Here's how the part is built. I have some questions about the finished solid (model axes, mm). Face numbers are marked on the shaded views. A direction names the side the tool comes from. Give positions to 0.01 mm unless a question says otherwise; leave off trailing zeros. Write each loop counter-clockwise with the first axis right and the second up, starting at its lowest first coordinate (ties: lowest second). Pieces come first, ordered by that corner, then holes. Notation, with made-up numbers: (19.25, 71.5) - (57.25, 71.5) arc R21 ccw to (57.25, 99.5) - close; hole circle Ø10 at (-32.75, -13). An arc over 180 degrees is marked (long way). Use a Markdown table: item, result.
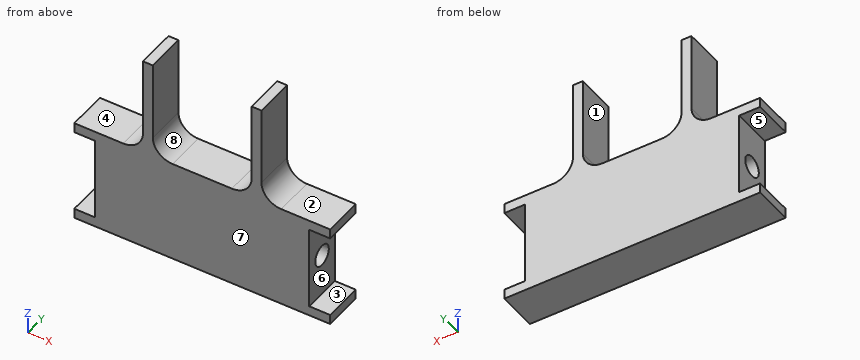
```python
from build123d import *

# Parameters (mm, degrees)
BOSS_EXTRUDE1_DEPTH = 12
SKETCH2_R           = 3.175
CUT_EXTRUDE1_DEPTH  = 79.871937341
SKETCH3_W           = 3
SKETCH3_H           = 12
BOSS_EXTRUDE2_DEPTH = 30
FILLET1_R           = 6


with BuildPart() as part:
    # Sketch1 → Boss-Extrude1 (new body)
    with BuildSketch(Plane(origin=(0, 0, 0), x_dir=(1, 0, 0), z_dir=(0, 1, 0))):
        Polygon((0, 0), (0, 3), (6.35, 3), (6.35, 28.4), (0, 28.4), (0, 31.4), (77.7, 31.4), (77.7, 28.4), (71.35, 28.4), (71.35, 3), (77.7, 3), (77.7, 0), align=None)
    extrude(amount=BOSS_EXTRUDE1_DEPTH)

    # Sketch2 → Cut-Extrude1 (cut, through all)
    with BuildSketch(Plane.ZY.offset(-6.35)):
        with Locations((-15.7, 6)):
            Circle(SKETCH2_R)
    extrude(amount=-CUT_EXTRUDE1_DEPTH, mode=Mode.SUBTRACT)

    # Sketch3 → Boss-Extrude2 (add)
    with BuildSketch(Plane.XY):
        with Locations((22.35, 6)):
            Rectangle(SKETCH3_W, SKETCH3_H)
        with Locations((55.35, 6)):
            Rectangle(SKETCH3_W, SKETCH3_H)
    extrude(amount=BOSS_EXTRUDE2_DEPTH)

    # Fillet1
    fillet1_edges = [part.edges().sort_by_distance(p)[0] for p in [
        (20.85, 6, 0),
        (53.85, 6, 0),
        (23.85, 6, 0),
        (56.85, 6, 0),
    ]]
    fillet(fillet1_edges, radius=FILLET1_R)


solid = part.part
```
Item 1: For the marked faces 1, 2, 3 and 4, which set-ups out of +Z, -Z, +X, -X, +Y, -Y let a thin tool reach every point of the face, with its end or its side?
Values:
| item | result |
|---|---|
| face 1 | +Z, +Y, -Y |
| face 2 | +Z, +X, +Y, -Y |
| face 3 | +X, +Y, -Y |
| face 4 | +Z, -X, +Y, -Y |
Item 2: If we section it at A-A, the plane y = 6: Write out the boundary of the cut face in (x, z) (3 decimals).
Values:
| item | result |
|---|---|
| outline | (0, -31.4) - (77.7, -31.4) - (77.7, -28.4) - (71.35, -28.4) - (71.35, -18.875) - (6.35, -18.875) - (6.35, -28.4) - (0, -28.4) - close; (0, -3) - (6.35, -3) - (6.35, -12.525) - (71.35, -12.525) - (71.35, -3) - (77.7, -3) - (77.7, 0) - (62.85, 0) arc R6 cw to (56.85, 6) - (56.85, 30) - (53.85, 30) - (53.85, 6) arc R6 cw to (47.85, 0) - (29.85, 0) arc R6 cw to (23.85, 6) - (23.85, 30) - (20.85, 30) - (20.85, 6) arc R6 cw to (14.85, 0) - (0, 0) - close |
Item 3: If we section it at D-D, the plane y = 1.75: Write out the boundary of the cut face in (x, z).
Values:
| item | result |
|---|---|
| outline | (0, -31.4) - (77.7, -31.4) - (77.7, -28.4) - (71.35, -28.4) - (71.35, -3) - (77.7, -3) - (77.7, 0) - (62.85, 0) arc R6 cw to (56.85, 6) - (56.85, 30) - (53.85, 30) - (53.85, 6) arc R6 cw to (47.85, 0) - (29.85, 0) arc R6 cw to (23.85, 6) - (23.85, 30) - (20.85, 30) - (20.85, 6) arc R6 cw to (14.85, 0) - (0, 0) - (0, -3) - (6.35, -3) - (6.35, -28.4) - (0, -28.4) - close |
Item 4: If we section it at C-C, the plane x = 37: Write out the boundary of the cut face in (y, z) (3 decimals), plus the area to 3 significant figures.
Values:
| item | result |
|---|---|
| outline | (0, -31.4) - (12, -31.4) - (12, 0) - (0, 0) - close; hole circle Ø6.35 at (6, -15.7) |
| area | 345 mm2 |
Item 5: Thinking about a two-plate mould opening in Z: for the marked faces 5, 6, 7 and 8, which applies, +Z half, -Z half, draft (parallel to the pull), parting line (faces both ways), or undercut?
Values:
| item | result |
|---|---|
| face 5 | undercut |
| face 6 | undercut |
| face 7 | draft |
| face 8 | +Z half |
Item 6: I need wall thicknesses on line 1 along X through (y, z) = (0.5, 16); line 2 along Z through (x, y) = (5.5, 9); line 3 along Y through (x, z) = (57.5, -15.7) (3 decimals). Which ranges of each line are inside material? Lowest first, please. Write a range as [from, to].
Values:
| item | result |
|---|---|
| line 1 | x = [20.85, 23.85], [53.85, 56.85] |
| line 2 | z = [-31.4, -28.4], [-3, 0] |
| line 3 | y = [0, 2.825], [9.175, 12] |
Item 7: If we section it at B-B, the plane z = 14.5: Write out the boundary of the cut face in (x, y).
Values:
| item | result |
|---|---|
| outline | (20.85, 0) - (23.85, 0) - (23.85, 12) - (20.85, 12) - close; (53.85, 0) - (56.85, 0) - (56.85, 12) - (53.85, 12) - close |
Item 8: Will these pins go through, and if not, where does the flat tip stop? pin 1 Ø6 at (y, z) = (6.5, 12) entering from +X; pin 2 Ø1.9 at (x, y) = (4.5, 8.5) entering from +Z; pin 3 Ø2 at (x, z) = (55, 18) entering from -Y; pin 4 Ø4 at (y, z) = (6, -15.7) entering from -X.
Values:
| item | result |
|---|---|
| pin 1 | stops at x = 56.85 |
| pin 2 | stops at z = 0 |
| pin 3 | stops at y = 0 |
| pin 4 | passes through |
